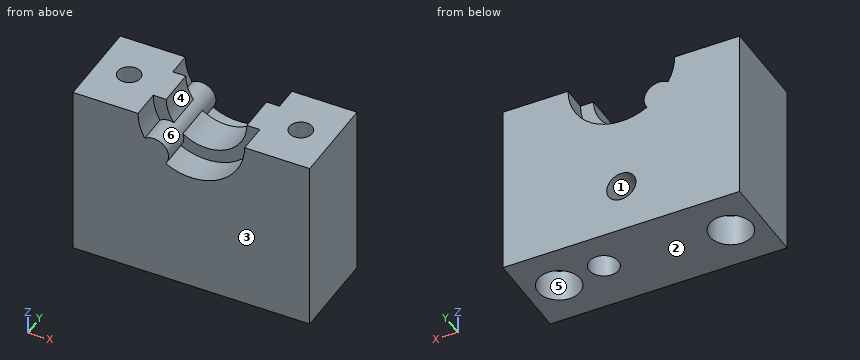
from build123d import *

# Parameters (mm, degrees)
SKETCH1_W                          = 36.4
SKETCH1_H                          = 14
BOSS_EXTRUDE1_DEPTH                = 27
CUT_EXTRUDE1_DEPTH                 = 14
BOSS_EXTRUDE2_START                = -3.7
BOSS_EXTRUDE2_DEPTH                = 5.8
SKETCH3_R                          = 1.75
CUT_EXTRUDE2_DEPTH                 = 27
SKETCH5_R                          = 3.25
CUT_EXTRUDE3_DEPTH                 = 5
SKETCH6_R                          = 2.25
HEAT_SET_INSERT_FOR_EXTRUDER_DEPTH = 7
SKETCH8_R                          = 2.25
CUT_EXTRUDE4_DEPTH                 = 4


with BuildPart() as part:
    # Sketch1 → Boss-Extrude1 (new body)
    with BuildSketch(Plane.XY):
        with Locations((18.2, 7)):
            Rectangle(SKETCH1_W, SKETCH1_H)
    extrude(amount=-BOSS_EXTRUDE1_DEPTH)

    # Sketch2 → Cut-Extrude1 (cut)
    with BuildSketch(Plane(origin=(0, 14, 0), x_dir=(1, 0, 0), z_dir=(0, 1, 0))):
        with BuildLine():
            ThreePointArc((11.019537046, 3.959918151), (10.258973737, 2.044529747), (10, 0))
            Line((10, 0), (26.4, 0))
            ThreePointArc((26.4, 0), (22.369452672, 7.060854369), (14.240081849, 7.180462954))
            ThreePointArc((14.240081849, 7.180462954), (14.028069991, 4.171930009), (11.019537046, 3.959918151))
        make_face()
    extrude(amount=-CUT_EXTRUDE1_DEPTH, mode=Mode.SUBTRACT)

    # Sketch4 → Boss-Extrude2 (add)
    with BuildSketch(Plane(origin=(0, 14, 0), x_dir=(1, 0, 0), z_dir=(0, 1, 0)).offset(BOSS_EXTRUDE2_START)):
        with BuildLine():
            Line((12, 0), (10, 0))
            ThreePointArc((10, 0), (18.2, 8.2), (26.4, 0))
            Line((26.4, 0), (24.4, 0))
            ThreePointArc((24.4, 0), (18.2, 6.2), (12, 0))
        make_face()
    extrude(amount=-BOSS_EXTRUDE2_DEPTH)

    # Sketch3 → Cut-Extrude2 (cut)
    with BuildSketch(Plane.XY):
        with Locations((5, 7)):
            Circle(SKETCH3_R)
        with Locations((31.4, 7)):
            Circle(SKETCH3_R)
    extrude(amount=-CUT_EXTRUDE2_DEPTH, mode=Mode.SUBTRACT)

    # Sketch5 → Cut-Extrude3 (cut)
    with BuildSketch(Plane(origin=(0, 0, -27), x_dir=(-1, 0, 0), z_dir=(0, 0, -1))):
        with Locations((-31.4, 7)):
            Circle(SKETCH5_R)
        with Locations((-5, 7)):
            Circle(SKETCH5_R)
    extrude(amount=-CUT_EXTRUDE3_DEPTH, mode=Mode.SUBTRACT)

    # Sketch6 → heat set insert for extruder (cut)
    with BuildSketch(Plane(origin=(0, 14, 0), x_dir=(1, 0, 0), z_dir=(0, 1, 0))):
        with Locations((18.2, 19.5)):
            Circle(SKETCH6_R)
    extrude(amount=-HEAT_SET_INSERT_FOR_EXTRUDER_DEPTH, mode=Mode.SUBTRACT)

    # Sketch8 → Cut-Extrude4 (cut)
    with BuildSketch(Plane(origin=(0, 0, -27), x_dir=(-1, 0, 0), z_dir=(0, 0, -1))):
        with Locations((-24, 8)):
            Circle(SKETCH8_R)
    extrude(amount=-CUT_EXTRUDE4_DEPTH, mode=Mode.SUBTRACT)


solid = part.part
CAD build for the part. Positions are in the model's coordinates, mm. Face numbers are marked on the shaded views. A direction names the side the tool comes from. Round coordinates to 2 decimals unless told otherwise and drop trailing zeros. Write each loop counter-clockwise with the first axis right and the second up, starting at its lowest first coordinate (ties: lowest second). Pieces come first, ordered by that corner, then holes.
(1) Probe line 1 along Y through (x, z) = (5, -13.5); line 2 along Y through (x, z) = (5, -24.55); line 3 along X through (y, z) = (6.25, -20.75). List the from-to ranges inside material, lowest first.
(2) Slice it at A-A, the plane y = 7.5. Count the separate pieces of the cut face and the enclosed holes in it, and give its area (3 significant figures).
(3) 3-axis set-ups, long thin cutter, end or side, ignore diameter. For the marked faces 4, 5 and 6: which of +Z, -Z, +X, -X, +Y, -Y reach the whole face in a straight line?
(4) Drop flat-ended pins along their axis: P1, Ø4, axis at x = 5, y = 7, coming from the -Z side; P2, Ø5, axis at x = 5, y = 7, coming from the +Z side; P3, Ø2.5, axis at x = 12, z = -1.5, coming from the -Y side; P4, Ø2, axis at x = 24, y = 8.5, coming from the -Z side. Give the stop position or say it passes through.
(5) Slice it at B-B, the plane x = 5. Write the cut outline in (y, z), and give its area (4 significant figures).
(6) Mould opens along Z. For the marked faces 1, 2 and 3 say: pulls with the +Z half, pulls with the -Z half, needs draft (parallel to the pull), parting line crosses it, or undercut.
(7) Slice it at C-C, the plane z = -11. Write the cut outline in (x, y).
(8) Slice it at D-D, the plane x = 18.2. Write the cut outline in (y, z), and give its area (3 significant figures).
From the geometry:
1. line 1: y = 0 to 5.25, 8.75 to 14
1. line 2: y = 0 to 3.75, 10.25 to 14
1. line 3: x = 0 to 3.42, 6.58 to 29.82, 32.98 to 36.4
2. separate pieces: 3
2. enclosed holes: 1
2. area: 678 mm2
3. face 4: +Z, +Y, -Y
3. face 5: -Z
3. face 6: none
4. P1: stops at z = -22
4. P2: stops at z = 0
4. P3: stops at y = 4.5
4. P4: stops at z = -23
5. outline: (0, -27) - (3.75, -27) - (3.75, -22) - (5.25, -22) - (5.25, 0) - (0, 0) - close; (8.75, -22) - (10.25, -22) - (10.25, -27) - (14, -27) - (14, 0) - (8.75, 0) - close
5. area: 268.5 mm2
6. face 1: undercut
6. face 2: pulls with the -Z half
6. face 3: needs draft
7. outline: (0, 0) - (36.4, 0) - (36.4, 14) - (0, 14) - close; hole circle Ø3.5 at (5, 7); hole circle Ø3.5 at (31.4, 7)
8. outline: (0, -27) - (14, -27) - (14, -21.75) - (7, -21.75) - (7, -17.25) - (14, -17.25) - (14, -8.2) - (10.3, -8.2) - (10.3, -6.2) - (4.5, -6.2) - (4.5, -8.2) - (0, -8.2) - close
8. area: 243 mm2
